Check sheet for the modelled part. Datum: model origin and axes. Units: mm. Round coordinates to 2 decimals unless told otherwise and drop trailing zeros. Loops run counter-clockwise (first coordinate to the right, second up) from the corner with the lowest first, then second, coordinate; pieces in that order, holes last. Notation, with made-up numbers: (-36, 88) -> (15, 88) arc R18 ccw to (15, 96) -> close; hole circle Ø7 at (-40, 32.25). An arc over 180 degrees is marked (long way). Return JSON: item names as keys, results as strings.
from build123d import *

# Parameters (mm, degrees)
F0_R     = 101.6
F0_R_2   = 25.4
F1_DEPTH = 6.35
F2_R     = 6.35
F3_DEPTH = 6.351


with BuildPart() as f1:
    # F0 (on Top) → F1 (new body)
    with BuildSketch(Plane.XY):
        Circle(F0_R)
        Circle(F0_R_2, mode=Mode.SUBTRACT)
    extrude(amount=F1_DEPTH)

    # F2 (on face) → F3 (cut, through all)
    with BuildSketch(Plane.XY.offset(6.35)):
        with Locations((0, 87.623763)):
            Circle(F2_R)
        with Locations((61.959357, 61.959357)):
            Circle(F2_R)
        with Locations((87.623763, 0)):
            Circle(F2_R)
    extrude(amount=-F3_DEPTH, mode=Mode.SUBTRACT)


solid = f1.part
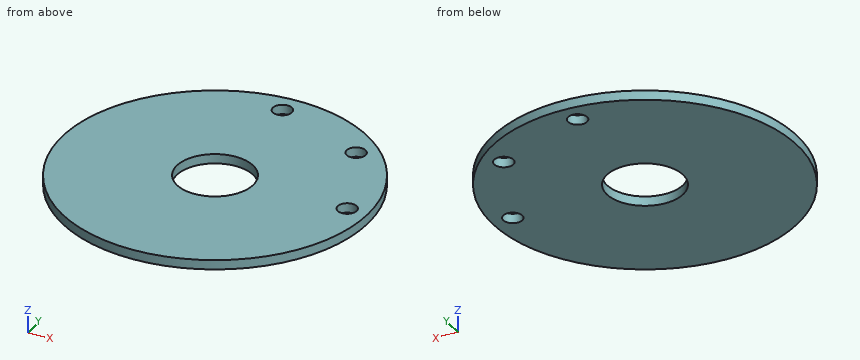
Q1. Section check A-A (y = 0). Record the boundary of the cut face in (x, z), then the cut area to 3 significant figures.
Results list:
{"outline": "(-101.6, 0) -> (-25.4, 0) -> (-25.4, 6.35) -> (-101.6, 6.35) -> close; (25.4, 0) -> (81.27, 0) -> (81.27, 6.35) -> (25.4, 6.35) -> close; (93.97, 0) -> (101.6, 0) -> (101.6, 6.35) -> (93.97, 6.35) -> close", "area": "887 mm^2"}
Q2. Section check D-D (x = -84). Record the boundary of the cut face in (y, z).
Results list:
{"outline": "(-57.15, 0) -> (57.15, 0) -> (57.15, 6.35) -> (-57.15, 6.35) -> close"}
Q3. Material ranges on line 1 (Y direction, x = 0, z = 4.75); line 2 (X direction, y = 90.5, z = 3); line 3 (Y direction, x = -5.5, z = 0.5), recorded low to high.
Results list:
{"line 1": "-101.6 to -25.4, 25.4 to 81.27, 93.97 to 101.6", "line 2": "-46.18 to -5.66, 5.66 to 46.18", "line 3": "-101.45 to -24.8, 24.8 to 84.45, 90.8 to 101.45"}
Q4. Section check C-C (z = 1). Record the boundary of the cut face in (x, y), then the cut area to 3 significant figures.
Results list:
{"outline": "circle Ø203.2 at (0, 0); hole circle Ø50.8 at (0, 0); hole circle Ø12.7 at (0, 87.62); hole circle Ø12.7 at (61.96, 61.96); hole circle Ø12.7 at (87.62, 0)", "area": "30,000 mm^2"}
Q5. Go/stop test with flat-tipped pins: pin 1 (1 mm diameter, centred on y = 54.5, z = 3.5, fed in from -X); pin 2 (2 mm diameter, centred on y = 72.5, z = 1.5, fed in from +X); pin 3 (3 mm diameter, centred on y = 19.5, z = 3.5, fed in from -X); pin 4 (12 mm diameter, centred on x = -72.5, y = 74.5, fed in from +Z). Record where each tip stops, or that it passes through.
Results list:
{"pin 1": "x = -86.06", "pin 2": "x = 72.18", "pin 3": "x = -99.99", "pin 4": "z = 6.35"}
